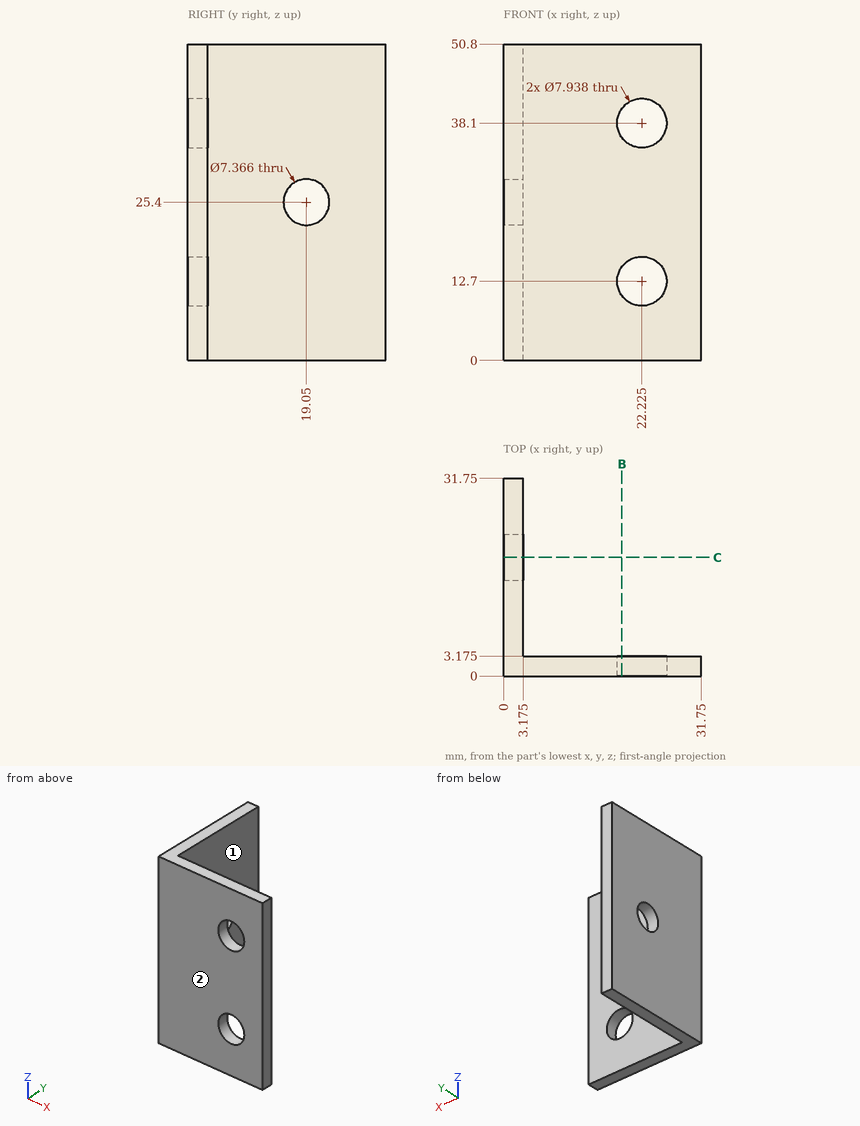
Can you work these out from the drawing? Everything is in mm from the part's minimum corner. A direction names the side the tool comes from. Coordinates: 2 decimals unless noted, no trailing zeros. Loops run counter-clockwise (first coordinate to the right, second up) from the corner with the lowest first, then second, coordinate; pieces in that order, holes last.
1) Please list where these lines run through material, in increasing order: line 1 along X through (y, z) = (1, 38); line 2 along X through (y, z) = (6, 21.5) (1 decimal).
Reported:
line 1: x = 0 to 18.26, 26.19 to 31.75
line 2: x = 0 to 3.2
2) Imagine slicing it at C-C (y = 19.05). List the corners of the cut face in (x, z) for me (1 decimal), and give its area (3 significant figures).
Reported:
outline: (0, 0) - (3.2, 0) - (3.2, 21.7) - (0, 21.7) - close; (0, 29.1) - (3.2, 29.1) - (3.2, 50.8) - (0, 50.8) - close
area: 138 mm2
3) Which directions (+Z, -Z, +X, -X, +Y, -Y) give clear straight access to the entire face, cutting with the end or side of a thin tool? Please do the marked faces 1 and 2.
Reported:
face 1: +Z, -Z, +X, +Y
face 2: +Z, -Z, +X, -X, -Y
4) Will these pins go through, and if not, where does the flat tip stop? pin 1 Ø6 at (x, z) = (8.5, 5.5) entering from +Y (1 decimal); pin 2 Ø10 at (y, z) = (26.5, 11.5) entering from +X (1 decimal).
Reported:
pin 1: stops at y = 3.2
pin 2: stops at x = 3.2
5) Imagine slicing it at B-B (x = 19). List the corners of the cut face in (y, z) for me (1 decimal).
Reported:
outline: (0, 0) - (3.2, 0) - (3.2, 10.4) - (0, 10.4) - close; (0, 15) - (3.2, 15) - (3.2, 35.8) - (0, 35.8) - close; (0, 40.4) - (3.2, 40.4) - (3.2, 50.8) - (0, 50.8) - close
